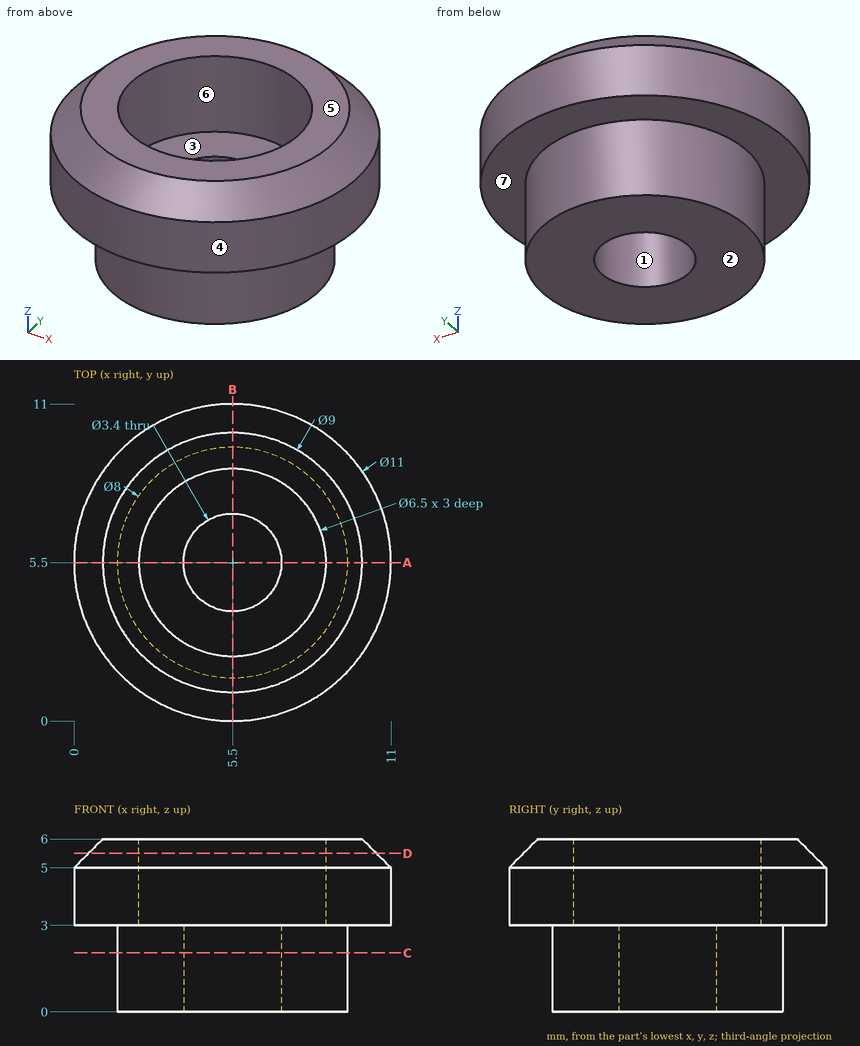
Verification items for this drawing (mm, ordinates from the low corner). A direction names the side the tool comes from. Give positions to 0.01 mm unless a question says otherwise; leave off trailing zeros. Write each loop counter-clockwise with the first axis right and the second up, starting at its lowest first coordinate (ties: lowest second). Pieces come first, ordered by that corner, then holes.
1) Section check A-A, the plane y = 5.5. Record the boundary of the cut face in (x, z).
2) Section check D-D, the plane z = 5.5. Record the boundary of the cut face in (x, y), and give its area (3 significant figures).
3) Section check C-C, the plane z = 2.05. Record the boundary of the cut face in (x, y), and give its area (3 significant figures).
4) Release check for a two-part mould opening along Y. For the marked faces 1, 2, 3 and 4 record: pulls with the +Y half, pulls with the -Y half, needs draft (parallel to the pull), parting line crosses it, or undercut.
5) Material ranges on L1, parallel to Y at x = 5.5, z = 2.25; L2, parallel to Z at x = 4.5, y = 2.75; L3, parallel to Y at x = 2.75, z = 5.3, recorded low to high.
6) Access from +Z, -Z, +X, -X, +Y, -Y to the whole of each face (thin tool, end or side, straight path). Record for the marked faces 5, 6 and 7.
7) Gauge pin test, flat ends, axial feed: pin 1 (2 mm diameter, centred on x = 4.5, y = 6, fed in from +Z); pin 2 (3.5 mm diameter, centred on x = 4, y = 3, fed in from -Z); pin 3 (2 mm diameter, centred on y = 4.5, z = 5.5, fed in from +X). Record the tip position at first contact, or that the pin passes through.
Computed:
1. outline: (0, 3) - (1.5, 3) - (1.5, 0) - (3.8, 0) - (3.8, 3) - (2.25, 3) - (2.25, 6) - (1, 6) - (0, 5) - close; (7.2, 0) - (9.5, 0) - (9.5, 3) - (11, 3) - (11, 5) - (10, 6) - (8.75, 6) - (8.75, 3) - (7.2, 3) - close
2. outline: circle Ø10 at (5.5, 5.5); hole circle Ø6.5 at (5.5, 5.5)
2. area: 45.4 mm2
3. outline: circle Ø8 at (5.5, 5.5); hole circle Ø3.4 at (5.5, 5.5)
3. area: 41.2 mm2
4. face 1: undercut
4. face 2: needs draft
4. face 3: undercut
4. face 4: parting line crosses it
5. L1: y = 1.5 to 3.8, 7.2 to 9.5
5. L2: z = 0 to 3
5. L3: y = 1.09 to 3.77, 7.23 to 9.91
6. face 5: +Z, +X, -X, +Y, -Y
6. face 6: +Z
6. face 7: -Z
7. pin 1: stops at z = 3
7. pin 2: stops at z = 0
7. pin 3: stops at x = 11
